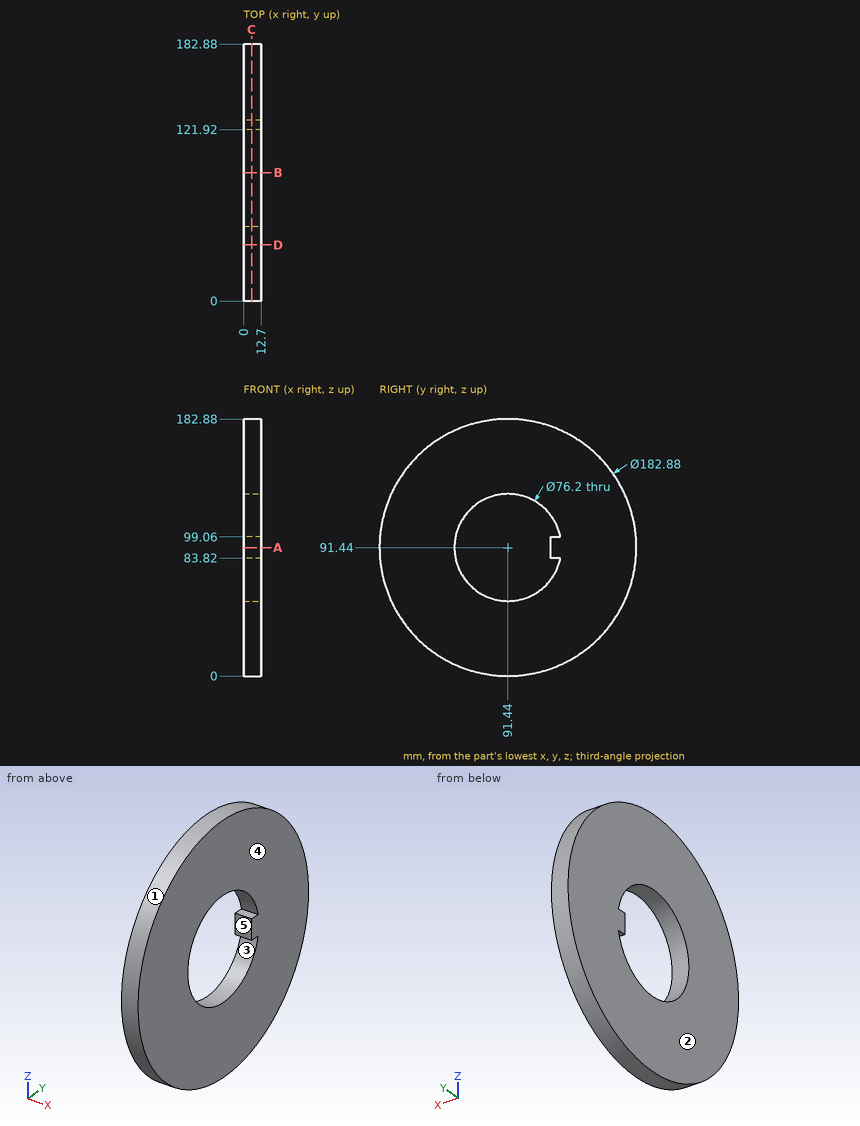
Here's the drawing with two shaded views (mm, measured from the low corner). I have some questions. A direction names the side the tool comes from. Coordinates: 2 decimals unless noted, no trailing zeros. Write each loop counter-clockwise with the first axis right and the second up, starting at its lowest first coordinate (ties: lowest second). Pieces come first, ordered by that corner, then holes. Notation, with made-up numbers: (-2.5, 15.25) -> (15.5, 15.25) arc R22 ccw to (15.5, 41.25) -> close; hole circle Ø6 at (-8, 87.5). An arc over 180 degrees is marked (long way). Answer as CSV lines item,"result".
1) If we section it at A-A on z = 91.44: Please give me the cut outline in (x, y).
Check result:
outline,"(0, 0) -> (12.7, 0) -> (12.7, 53.34) -> (0, 53.34) -> close; (0, 121.92) -> (12.7, 121.92) -> (12.7, 182.88) -> (0, 182.88) -> close"
2) If we section it at C-C on x = 5.75: Please give me the cut outline in (y, z).
Check result:
outline,"circle Ø182.88 at (91.44, 91.44); hole (121.92, 83.82) -> (121.92, 99.06) -> (128.77, 99.06) arc R38.1 ccw (long way) to (128.77, 83.82) -> close"
3) If we section it at B-B on y = 91.44: Please give me the cut outline in (x, z).
Check result:
outline,"(0, 0) -> (12.7, 0) -> (12.7, 53.34) -> (0, 53.34) -> close; (0, 129.54) -> (12.7, 129.54) -> (12.7, 182.88) -> (0, 182.88) -> close"
4) If we section it at D-D on y = 40: Please give me the cut outline in (x, z), then the cut area to 3 significant figures.
Check result:
outline,"(0, 15.84) -> (12.7, 15.84) -> (12.7, 167.04) -> (0, 167.04) -> close"
area,"1,920 mm²"
5) On a 3-axis mill with a long thin cutter (end or side, diameter ignored), from which of +Z, -Z, +X, -X, +Y, -Y can I reach the whole of each face in a straight line? I mean the marked faces 4 and 5. Say none if no direction works.
Check result:
face 4,"+Z, -Z, +X, +Y, -Y"
face 5,"+X, -X"
6) If we mould it in two halves opening along Z, with no side actions, what happens to the marked faces 1, 2 and 3? For each: +Z half, -Z half, draft (parallel to the pull), parting line (faces both ways), or undercut.
Check result:
face 1,"parting line"
face 2,"draft"
face 3,"undercut"
7) If I drill on line 1 (Y direction, x = 9, z = 91.44); line 2 (Z direction, x = 8, y = 122); line 3 (Y direction, x = 3.25, z = 64), over which ranges is the centre line in solid material (lowest first)? Write a range as from..to.
Check result:
line 1,"0..53.34, 121.92..182.88"
line 2,"5.26..68.69, 83.82..99.06, 114.19..177.62"
line 3,"4.21..65.01, 117.87..178.67"
8) Will these pins go through, and if not, where does the flat tip stop? P1, Ø5.5, axis at x = 4, y = 126, coming from the -Z side; P2, Ø3, axis at x = 8, y = 116.5, coming from the +Z side; P3, Ø1, axis at x = 3, y = 126, coming from the -Z side.
Check result:
P1,"z = 5.71"
P2,"z = 179.79"
P3,"z = 6.58"
